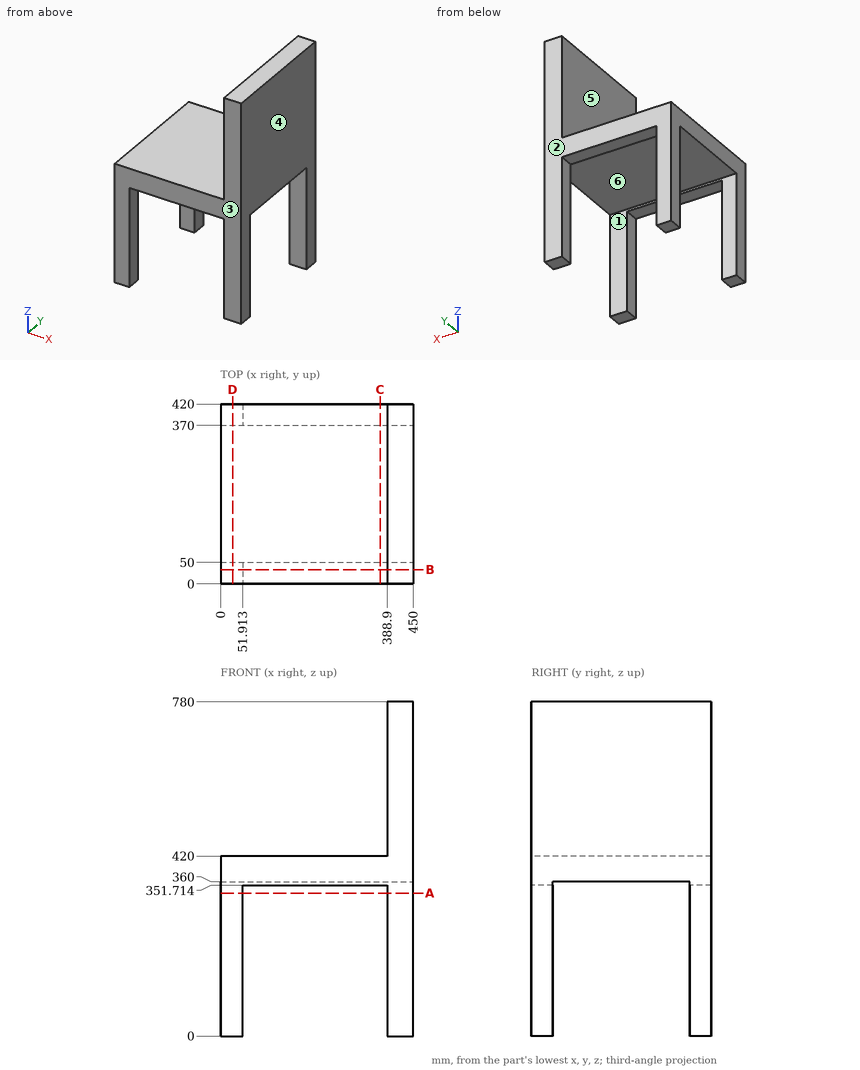
Print and shaded views of the part. All mm, measured from the part's lowest x, y and z. A direction names the side the tool comes from. Give positions to 0.01 mm unless a question says otherwise; leave off trailing zeros. Order: outer loops, then holes, each group sorted by start corner. A loop starts at its lowest first (then second) coordinate and runs counter-clockwise, first axis right, second up. Notation, with made-up numbers: (25, 28) -> (41, 28) arc R22 ccw to (41, 50) -> close; hole circle Ø9 at (-3, 33). An arc over 180 degrees is marked (long way). Use CSV: the item, a comma, the result in double quotes.
1. Band-saw the part on A-A, the plane z = 333.5. Give the cut face in (x, y), then the cut area to 3 significant figures.
Outcome:
outline,"(0, 0) -> (51.91, 0) -> (51.91, 50) -> (0, 50) -> close; (0, 370) -> (51.91, 370) -> (51.91, 420) -> (0, 420) -> close; (388.9, 0) -> (450, 0) -> (450, 50) -> (388.9, 50) -> close; (388.9, 370) -> (450, 370) -> (450, 420) -> (388.9, 420) -> close"
area,"11,300 mm²"
2. Mould opens along Y. For the marked faces 1, 2 and 3 say: +Y half, -Y half, draft (parallel to the pull), parting line (faces both ways), or undercut.
Outcome:
face 1,"undercut"
face 2,"+Y half"
face 3,"-Y half"
3. Band-saw the part on B-B, the plane y = 33.5. Give the cut face in (x, z).
Outcome:
outline,"(0, 0) -> (51.91, 0) -> (51.91, 351.71) -> (388.9, 351.71) -> (388.9, 0) -> (450, 0) -> (450, 780) -> (388.9, 780) -> (388.9, 420) -> (0, 420) -> close"
4. 3-axis set-ups, long thin cutter, end or side, ignore diameter. For the marked faces 4, 5 and 6: which of +Z, -Z, +X, -X, +Y, -Y reach the whole face in a straight line?
Outcome:
face 4,"+Z, -Z, +X, +Y, -Y"
face 5,"+Z, -X, +Y, -Y"
face 6,"-Z, +X, -X"
5. Drop flat-ended pins along their axis: pin 1 (1 mm diameter, centred on x = 238, y = 257.5, fed in from +Z); pin 2 (15 mm diameter, centred on x = 143, y = 383.5, fed in from -Z); pin 3 (12 mm diameter, centred on y = 255.5, z = 560, fed in from -X). Give the stop position or say it passes through.
Outcome:
pin 1,"z = 420"
pin 2,"z = 351.71"
pin 3,"x = 388.9"
6. Band-saw the part on C-C, the plane x = 372.5. Give the cut face in (y, z).
Outcome:
outline,"(0, 351.71) -> (50, 351.71) -> (50, 360) -> (370, 360) -> (370, 351.71) -> (420, 351.71) -> (420, 420) -> (0, 420) -> close"
7. Drill centre lines: line 1 along Z through (x, y) = (176.5, 278); line 2 along X through (y, z) = (284, 737); line 3 along Z through (x, y) = (400, 283). Where is each one in solid material? Low to high. Write a range as from..to.
Outcome:
line 1,"360..420"
line 2,"388.9..450"
line 3,"360..780"
8. Band-saw the part on D-D, the plane x = 28. Give the cut face in (y, z).
Outcome:
outline,"(0, 0) -> (50, 0) -> (50, 360) -> (370, 360) -> (370, 0) -> (420, 0) -> (420, 420) -> (0, 420) -> close"
